Could you check a few things on this drawing? It's one solid part, dimensions in mm from its lowest x, y, z. A direction names the side the tool comes from. Coordinates: 2 decimals unless noted, no trailing zeros. Order: outer loops, then holes, each group sorted by start corner. A loop starts at its lowest first (then second) coordinate and runs counter-clockwise, first axis right, second up.
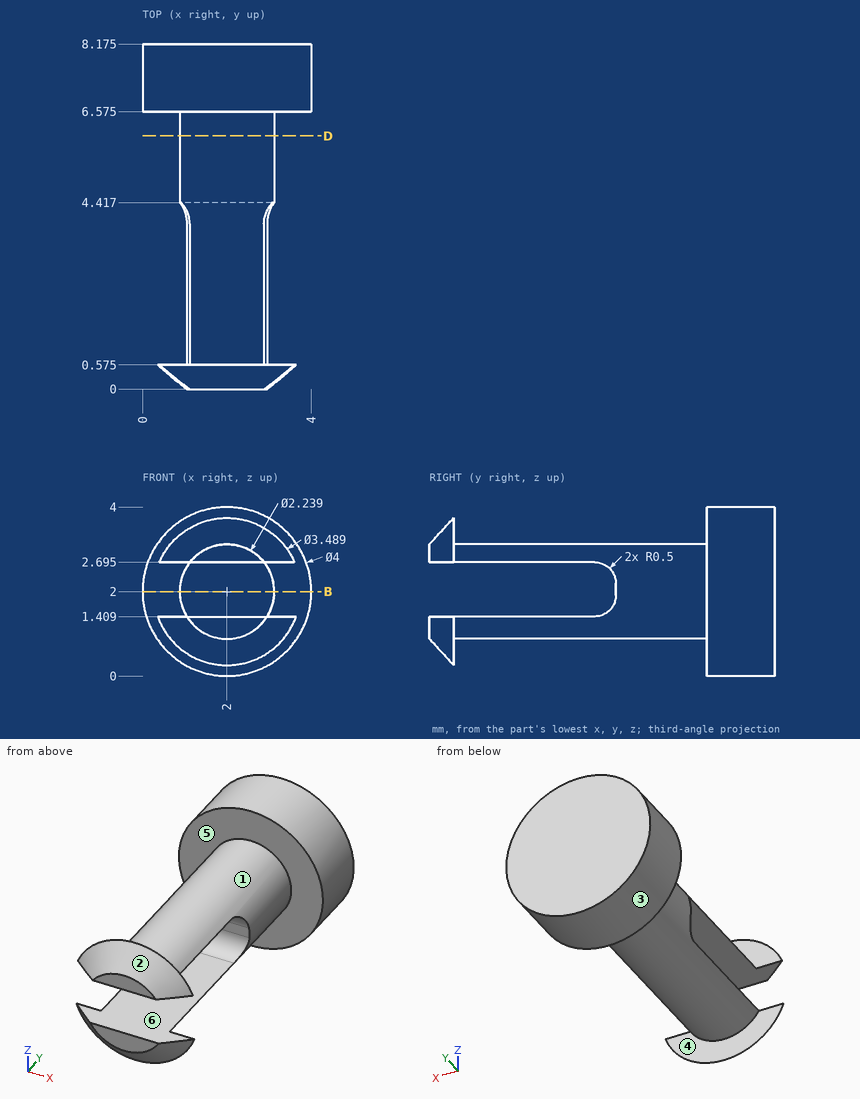
1. Imagine slicing it at B-B on z = 2. Please give me the cut outline in (x, y) (1 decimal), then the cut area to 3 significant figures.
Completed:
outline: (0, 6.6) - (0.9, 6.6) - (0.9, 4.4) - (3.1, 4.4) - (3.1, 6.6) - (4, 6.6) - (4, 8.2) - (0, 8.2) - close
area: 11.2 mm2
2. Thinking about a two-plate mould opening in Y: for the marked faces 1, 2 and 3, which applies, pulls with the +Y half, pulls with the -Y half, needs draft (parallel to the pull), parting line crosses it, or undercut?
Completed:
face 1: undercut
face 2: pulls with the -Y half
face 3: needs draft
3. I'm going to push flat-ended pins straight in: pin 1 (2 mm diameter, centred on x = 3, y = 2.5, fed in from +Z); pin 2 (1 mm diameter, centred on x = 2, y = 1.5, fed in from -Z); pin 3 (1.5 mm diameter, centred on x = 0.5, y = 4, fed in from -Z). Where does each tip first touch, or does it pass through?
Completed:
pin 1: stops at z = 3.12
pin 2: stops at z = 0.88
pin 3: stops at z = 1.17
4. Please list where these lines run through material, in increasing order: probe 1 along Z at (x, y) = (1.95, 3) (1 decimal); probe 2 along Y at (x, z) = (2.7, 3.35) (1 decimal); probe 3 along Y at (x, z) = (0.4, 1.9) (1 decimal).
Completed:
probe 1: z = 0.9 to 1.4, 2.7 to 3.1
probe 2: y = 0.4 to 0.6, 6.6 to 8.2
probe 3: y = 6.6 to 8.2
5. On a 3-axis mill with a long thin cutter (end or side, diameter ignored), from which of +Z, -Z, +X, -X, +Y, -Y can I reach the whole of each face in a straight line? I mean the marked faces 4, 5 and 6. Say none if no direction works.
Completed:
face 4: -Z
face 5: none
face 6: +X, -X, -Y
6. Imagine slicing it at D-D on y = 6. Please give me the cut outline in (x, z).
Completed:
outline: circle Ø2.24 at (2, 2)
